Autodesk Inventor part; units mm, degrees
ref_plane "YZ Plane" through (0, 0, 0) normal (1, 0, 0) x (0, 1, 0)
ref_plane "XZ Plane" through (0, 0, 0) normal (0, 1, 0) x (-1, 0, 0)
ref_plane "XY Plane" through (0, 0, 0) normal (0, 0, 1) x (1, 0, 0)
sketch "Sketch2" plane through (0, 0, 0) normal (1, 0, 0) x (0, 1, 0)
  circle A0 centre (0, 0) radius 1.25
  dimension "d8" = 2.5
extrude "Extrusion1" add sketch "Sketch2" along normal blind 14
sketch "Sketch6" plane through (0, 0, 0) normal (0, 0, 1) x (1, 0, 0)
  line L0 (14, -1.25) -> (14, 1.25)
  line L1 (14, 0) -> (14, 0.125)
  line L2 (14, 0.125) -> (15.875, 0.125)
  line L3 (16, 0) -> (16, -11.875)
  line L4 (14, 0) -> (15.875, 0)
  line L5 (15.875, 0) -> (15.875, -11.875)
  line L6 (15.875, -11.875) -> (16, -11.875)
  line L7 (15.875, 0) -> (16, 0)
  line L8 (17.9417, 0) -> (15.75, 0)
  arc A0 (15.875, -0.125) -> (15.75, 0) centre (15.75, -0.125) ccw
  line L9 (15.75, 0) -> (16, 0)
  line L10 (0, 0) -> (0, 0.125)
  line L11 (0, 0.125) -> (-1.875, 0.125)
  line L12 (-2, 0) -> (-2, -11.875)
  line L13 (-2, -11.875) -> (-1.875, -11.875)
  line L14 (-1.875, -11.875) -> (-1.875, -0.125)
  line L15 (-1.75, 0) -> (0, 0)
  arc A1 (-1.875, 0.125) -> (-2, 0) centre (-1.875, 0) ccw
  arc A2 (-1.75, 0) -> (-1.875, -0.125) centre (-1.75, -0.125) ccw
  line L16 (-1.75, 0) -> (-2, 0)
  line L17 (-1.875, -0.125) -> (-1.875, 0)
  arc A3 (16, 0) -> (15.875, 0.125) centre (15.875, 0) ccw
  point P0 (16, 0.125)
  point P1 (18.875, 0.125)
  point P2 (-2, 0.125)
  point P3 (-1.875, 0)
  dimension "d16" = 0.125
  dimension "d17" = 2
  dimension "d18" = 12
  dimension "d19" = 1.875
  dimension "d26" = 0.125
  dimension "d27" = 2
  dimension "d28" = 0.125
  dimension "d29" = 0.125
  dimension "d30" = 0.125
  dimension "d33" = 0.125
  dimension "d35" = 12
revolve "Revolution2" add sketch "Sketch6" angle 360 about axis through (14, 0, 0) along (1, 0, 0) contours L0 L2 A3 L7 L4
revolve "Revolution3" add sketch "Sketch6" angle 360 about axis through (15.875, 0, 0) along (0, -1, 0) contours L7 L3 L6 L5
revolve "Revolution4" add sketch "Sketch6" angle 360 about axis through (-1.75, 0, 0) along (1, 0, 0) contours L15 L16 A1 L11 L10
revolve "Revolution5" add sketch "Sketch6" angle 360 about axis through (-1.875, -11.875, 0) along (0, 1, 0) contours L14 L13 L12 L16 L17
equation "\"d35\" = d18"
properties part number "Reed Switch Puerta Derecha" material "Aluminum 6061"
The model under review builds one solid part; all positions refer to its coordinate system, in mm. Round coordinates to 2 decimals unless told otherwise and drop trailing zeros. Loops run counter-clockwise (first coordinate to the right, second up) from the corner with the lowest first, then second, coordinate; pieces in that order, holes last. Notation, with made-up numbers: (26.25, -27) -> (36.25, -27) arc R9 ccw to (36.25, -14) -> close; hole circle Ø9 at (67, 67). An arc over 180 degrees is marked (long way). Write item = value, one per line. Start each with the question number.
Item 1: Take a section at C-C on z = 0.8. Give the boundary of the cut face in (x, y), plus the area to 3 significant figures.
Item 2: Take a section at A-A on y = -2.25. Give the boundary of the cut face in (x, z) (3 decimals), plus the area to 3 significant figures.
Item 3: To check wall thickness, follow L1, parallel to Y at x = 8.25, z = -0.05; L2, parallel to Z at x = -0.5, y = 0 (3 decimals); L3, parallel to X at y = -0.75, z = 0.5. State the ranges of each line that lie inside material, in increasing order.
Item 4: Take a section at B-B on x = 3. Give the boundary of the cut face in (y, z).
Result:
q1.outline = (0, -0.96) -> (14, -0.96) -> (14, 0.96) -> (0, 0.96) -> close
q1.area = 26.9 mm²
q2.outline = circle Ø0.25 at (-1.875, 0); circle Ø0.25 at (15.875, 0)
q2.area = 0.0982 mm²
q3.L1 = -1.25 to 1.25
q3.L2 = -0.125 to 0.125
q3.L3 = 0 to 14
q4.outline = circle Ø2.5 at (0, 0)
